```python
from build123d import *
from OCP.BRepFilletAPI import BRepFilletAPI_MakeChamfer

# Parameters (mm, degrees)
SKETCH1_W             = 20
SKETCH1_H             = 81.5
SKETCH1_R             = 1.5
SKETCH1_H_2           = 20
BOSS_EXTRUDE1_DEPTH   = 20
CHAMFER1_SIZE         = 2.5
SKETCH2_W             = 20
SKETCH2_H             = 7
CUT_EXTRUDE1_DEPTH    = 65
CHAMFER2_SIZE         = 2.5
CUT_EXTRUDE2_DEPTH    = 1.57
CHAMFER3_SIZE         = 2.5
SKETCH4_W             = 12
SKETCH4_H             = 23.86
CUT_EXTRUDE3_DEPTH    = 15.13
CUT_EXTRUDE4_DEPTH    = 94.547528027
SKETCH6_R             = 2.77
CUT_EXTRUDE5_DEPTH    = 95.192621792
CUT_EXTRUDE6_DEPTH    = 95.192621792
CHAMFER8_SIZE         = 1
CHAMFER8_SIZE2        = 1.129384369
CUT_EXTRUDE7_DEPTH    = 92.006867873
CHAMFER9_SIZE         = 1
CHAMFER9_SIZE2        = 1.129384369
CHAMFER9_EDGE_2_SIZE  = 1
CHAMFER9_EDGE_2_SIZE2 = 1.129384369
CHAMFER9_EDGE_3_SIZE  = 1
CHAMFER9_EDGE_3_SIZE2 = 1.129384369


with BuildPart() as part:
    # Sketch1 → Boss-Extrude1 (new body)
    # profile 1 of 2: a face of its own
    with BuildSketch(Plane.XY):
        with Locations((0, -50.75)):
            Rectangle(SKETCH1_W, SKETCH1_H)
        with Locations((0, -81.5)):
            Circle(SKETCH1_R, mode=Mode.SUBTRACT)
    # profile 2 of 2: a face of its own
    with BuildSketch(Plane.XY):
        Rectangle(SKETCH1_W, SKETCH1_H_2)
    extrude(amount=BOSS_EXTRUDE1_DEPTH)

    # Chamfer1
    chamfer1_edges = [part.edges().sort_by_distance(p)[0] for p in [
        (0, -91.5, 20),
        (-10, -91.5, 10),
        (-10, 10, 10),
        (10, 10, 10),
        (10, -91.5, 10),
        (10, -40.75, 20),
        (-10, -40.75, 20),
        (0, -91.5, 0),
    ]]
    chamfer(chamfer1_edges, length=CHAMFER1_SIZE)

    # Sketch2 → Cut-Extrude1 (cut)
    with BuildSketch(Plane.XZ.offset(91.5)):
        with Locations((0, 12.5)):
            Rectangle(SKETCH2_W, SKETCH2_H)
    extrude(amount=-CUT_EXTRUDE1_DEPTH, mode=Mode.SUBTRACT)

    # Chamfer2
    chamfer2_edges = [part.edges().sort_by_distance(p)[0] for p in [
        (10, -26.5, 12.5),
        (-10, -26.5, 12.5),
    ]]
    chamfer(chamfer2_edges, length=CHAMFER2_SIZE)

    # Sketch3 → Cut-Extrude2 (cut)
    with BuildSketch(Plane.XY.offset(20)):
        Polygon((0, -19.84), (0, -14), (0, 3.96), (0, 8.09), (-6, 8.09), (-6, -23.97), (0, -23.97), align=None)
        Polygon((0, 3.96), (0, -14), (0, -19.84), (0, -23.97), (6, -23.97), (6, 8.09), (0, 8.09), align=None)
    extrude(amount=-CUT_EXTRUDE2_DEPTH, mode=Mode.SUBTRACT)

    # Chamfer3
    # the kernel refuses this chamfer: 2.5 mm, written as the material it takes off along each edge
    with BuildSketch(Plane(origin=(13.92920747, 10, 20), x_dir=(0, -0.9996219169112968, 0.027495876610586317), z_dir=(-1, 0, 0))) as chamfer3_piece_1:
        Polygon((CHAMFER3_SIZE * 0.999621916911, -CHAMFER3_SIZE * 0.0274958766106), (-CHAMFER3_SIZE * 0.0274958766106, -CHAMFER3_SIZE * 0.999621916911), (0, 0), align=None)
    extrude(amount=27.85841494, mode=Mode.SUBTRACT)

    # Sketch4 → Cut-Extrude3 (cut)
    with BuildSketch(Plane.XY.offset(18.43)):
        with Locations((0, -7.94)):
            Rectangle(SKETCH4_W, SKETCH4_H)
    extrude(amount=-CUT_EXTRUDE3_DEPTH, mode=Mode.SUBTRACT)

    # Sketch5 → Cut-Extrude4 (cut, through all)
    with BuildSketch(Plane.XY.offset(3.3)):
        Polygon((0, -19.87), (4.5, -19.87), (4.5, -16.37), (0, -16.37), (-4.5, -16.37), (-4.5, -19.87), align=None)
    extrude(amount=-CUT_EXTRUDE4_DEPTH, mode=Mode.SUBTRACT)

    # Sketch6 → Cut-Extrude5 (cut, through all)
    with BuildSketch(Plane(origin=(0, 0, 0), x_dir=(-1, 0, 0), z_dir=(0, 0, -1))):
        Circle(SKETCH6_R)
    extrude(amount=-CUT_EXTRUDE5_DEPTH, mode=Mode.SUBTRACT)

    # Sketch7 → Cut-Extrude6 (cut, through all)
    with BuildSketch(Plane.XY.offset(20)):
        Polygon((-5, -86.5), (-7.5, -63.625), (-7.5, -89), (7.5, -89), (7.5, -63.625), (5, -86.5), align=None)
        Polygon((-7.5, -63.625), (-10, -40.75), (-10, -91.5), (10, -91.5), (10, -40.75), (7.5, -63.625), (7.5, -89), (-7.5, -89), align=None)
    extrude(amount=-CUT_EXTRUDE6_DEPTH, mode=Mode.SUBTRACT)

    # Chamfer8: one chamfer whose edges measure the first distance from different faces: ONE call of the kernel's chamfer builder (chamfer() names one face for all edges)
    chamfer8_edges_1 = [part.edges().sort_by_distance(p)[0] for p in [
        (-5, -86.5, 18),
    ]]
    chamfer8_side_1 = [part.faces().sort_by_distance(p)[0] for p in [
        (0, -86.5, 18),
    ]]
    chamfer8_edges_2 = [part.edges().sort_by_distance(p)[0] for p in [
        (0, -86.5, 20),
    ]]
    chamfer8_edges_3 = [part.edges().sort_by_distance(p)[0] for p in [
        (5, -86.5, 18),
    ]]
    chamfer8_side_3 = [part.faces().sort_by_distance(p)[0] for p in [
        (7.191358025, -66.449074074, 17.783950617),
    ]]
    chamfer8 = BRepFilletAPI_MakeChamfer(part.part.solid().wrapped)
    for e in chamfer8_edges_1:
        chamfer8.Add(CHAMFER8_SIZE, CHAMFER8_SIZE2, e.wrapped, chamfer8_side_1[0].wrapped)  # the first distance lies on this face
    for e in chamfer8_edges_2:
        chamfer8.Add(CHAMFER8_SIZE, e.wrapped)
    for e in chamfer8_edges_3:
        chamfer8.Add(CHAMFER8_SIZE, CHAMFER8_SIZE2, e.wrapped, chamfer8_side_3[0].wrapped)  # the first distance lies on this face
    add(Compound.cast(chamfer8.Shape()), mode=Mode.REPLACE)

    # Sketch8 → Cut-Extrude7 (cut, through all)
    with BuildSketch(Plane.ZY.offset(10)):
        Polygon((0, -40.75), (5, -86.5), (0, -86.5), align=None)
    extrude(amount=-CUT_EXTRUDE7_DEPTH, mode=Mode.SUBTRACT)

    # Chamfer9
    chamfer9_edges = [part.edges().sort_by_distance(p)[0] for p in [
        (-5, -86.5, 7),
    ]]
    chamfer9_side = [part.faces().sort_by_distance(p)[0] for p in [
        (0, -86.5, 7),
    ]]
    chamfer(chamfer9_edges, length=CHAMFER9_SIZE, length2=CHAMFER9_SIZE2, reference=chamfer9_side[0])

    # Chamfer9 edge 2
    chamfer9_edge_2_edges = [part.edges().sort_by_distance(p)[0] for p in [
        (5, -86.5, 7),
    ]]
    chamfer9_edge_2_side = [part.faces().sort_by_distance(p)[0] for p in [
        (0, -86.5, 7),
    ]]
    chamfer(chamfer9_edge_2_edges, length=CHAMFER9_EDGE_2_SIZE, length2=CHAMFER9_EDGE_2_SIZE2, reference=chamfer9_edge_2_side[0])

    # Chamfer9 edge 3
    chamfer9_edge_3_edges = [part.edges().sort_by_distance(p)[0] for p in [
        (0, -86.5, 5),
    ]]
    chamfer9_edge_3_side = [part.faces().sort_by_distance(p)[0] for p in [
        (0, -86.5, 7),
    ]]
    chamfer(chamfer9_edge_3_edges, length=CHAMFER9_EDGE_3_SIZE, length2=CHAMFER9_EDGE_3_SIZE2, reference=chamfer9_edge_3_side[0])


solid = part.part
```
Geometry check sheet. Reference: the model listing, model coordinates, mm. A direction names the side the tool comes from. Coordinates: 2 decimals unless noted, no trailing zeros. Loops run counter-clockwise (first coordinate to the right, second up) from the corner with the lowest first, then second, coordinate; pieces in that order, holes last.
Item 1: Access from +Z, -Z, +X, -X, +Y, -Y to the whole of each face (thin tool, end or side, straight path). Record for faces 5 (the face through (0, -19.87, 9)), 6 (the face through (0, -26.5, 13)), 7 (the face through (-4.5, -18, 2)).
Item 2: Release check for a two-part mould opening along X. For faces 1 (the face through (8.137, -57.793, 5.563)), 2 (the face through (0, -86.5, 18)), 3 (the face through (0, -22, 18.43)), 4 (the face through (-6, -8, 12)) record: released by +X, released by -X, zero draft, split by the parting line, or undercut.
Item 3: Thickness scan on line 1 (Y direction, x = 0, z = 7.4); line 2 (Z direction, x = -6.75, y = -35); line 3 (Y direction, x = 1.25, z = 17). Record the ranges inside material, lowest first.
Item 4: Sectioned sample at B-B, the plane z = 12. Record the boundary of the cut face in (x, y).
Item 5: Sectioned sample at D-D, the plane y = -5. Record the boundary of the cut face in (x, z).
Item 6: Go/stop test with flat-tipped pins: pin 1 Ø6 at (x, y) = (1.5, -8) entering from +Z; pin 2 Ø0.8 at (x, z) = (-3, 19) entering from +Y; pin 3 Ø1.5 at (y, z) = (-62, 3) entering from -X; pin 4 Ø2.5 at (x, y) = (0, -81.5) entering from +Z. Record where each tip stops, or that it passes through.
Item 7: Sectioned sample at A-A, the plane y = -17.5. Record the boundary of the cut face in (x, z), then the cut area to 3 significant figures.
Item 8: Sectioned sample at C-C, the plane x = 0. Count the separate pieces of the cut face and the enclosed holes in it, then the cut area to 3 significant figures.
Check result:
1. face 5: +Z
1. face 6: +X, -X, -Y
1. face 7: +Z, -Z
2. face 1: released by +X
2. face 2: zero draft
2. face 3: undercut
2. face 4: undercut
3. line 1: y = -86.5 to -83, -80 to -19.87, 3.99 to 10
3. line 2: z = 0 to 9, 16 to 20
3. line 3: y = -86.5 to -82.33, -80.67 to -19.87, 3.99 to 10
4. outline: (-10, -24) - (-7.5, -26.5) - (7.5, -26.5) - (10, -24) - (10, 7.5) - (7.5, 10) - (-7.5, 10) - (-10, 7.5) - close; hole (-6, -19.87) - (6, -19.87) - (6, 3.99) - (-6, 3.99) - close
5. outline: (-10, 0) - (10, 0) - (10, 17.5) - (7.5, 20) - (6, 20) - (6, 3.3) - (-6, 3.3) - (-6, 20) - (-7.5, 20) - (-10, 17.5) - close
6. pin 1: stops at z = 3.3
6. pin 2: stops at y = 8.9
6. pin 3: stops at x = -7.76
6. pin 4: passes through
7. outline: (-10, 0) - (-4.5, 0) - (-4.5, 3.3) - (-6, 3.3) - (-6, 20) - (-7.5, 20) - (-10, 17.5) - close; (4.5, 0) - (10, 0) - (10, 17.5) - (7.5, 20) - (6, 20) - (6, 3.3) - (4.5, 3.3) - close
7. area: 164 mm2
8. separate pieces: 5
8. enclosed holes: 0
8. area: 925 mm2
